```python
from build123d import *

# Parameters (mm, degrees)
PAD_DEPTH       = 41
SKETCH001_W     = 25
SKETCH001_H     = 50
POCKET_DEPTH    = 44.001
SKETCH002_W     = 45
SKETCH002_H     = 10
POCKET001_DEPTH = 30.001
SKETCH003_R     = 12
SKETCH003_R_2   = 1.625
POCKET002_DEPTH = 30.001
SKETCH004_R     = 2.75
POCKET003_DEPTH = 6.001
CHAMFER_SIZE    = 0.5
CHAMFER001_SIZE = 0.5
CHAMFER002_SIZE = 0.25


with BuildPart() as part:
    # Sketch → Pad (new body, symmetric)
    with BuildSketch(Plane.YZ):
        Polygon((0, 44), (0, 0), (-30, 0), (-30, 6), (-6, 44), align=None)
    extrude(amount=PAD_DEPTH, both=True)

    # Sketch001 → Pocket (cut, through all)
    with BuildSketch(Plane.YX):
        with Locations((-18.5, 0)):
            Rectangle(SKETCH001_W, SKETCH001_H)
    extrude(amount=-POCKET_DEPTH, mode=Mode.SUBTRACT)

    # Sketch002 → Pocket001 (cut, through all)
    with BuildSketch(Plane.ZX):
        with Locations((28.5, 36)):
            Rectangle(SKETCH002_W, SKETCH002_H)
        with Locations((28.5, -36)):
            Rectangle(SKETCH002_W, SKETCH002_H)
    extrude(amount=-POCKET001_DEPTH, mode=Mode.SUBTRACT)

    # Sketch003 → Pocket002 (cut, through all)
    with BuildSketch(Plane.ZX):
        with Locations((22, 0)):
            Circle(SKETCH003_R)
        with Locations((6.5, 15.5)):
            Circle(SKETCH003_R_2)
        with Locations((37.5, 15.5)):
            Circle(SKETCH003_R_2)
        with Locations((6.5, -15.5)):
            Circle(SKETCH003_R_2)
        with Locations((37.5, -15.5)):
            Circle(SKETCH003_R_2)
    extrude(amount=-POCKET002_DEPTH, mode=Mode.SUBTRACT)

    # Sketch004 → Pocket003 (cut, through all)
    with BuildSketch(Plane(origin=(0, 0, 6), x_dir=(0, -1, 0), z_dir=(0, 0, 1))):
        with Locations((5, 36)):
            Circle(SKETCH004_R)
        with Locations((25, 36)):
            Circle(SKETCH004_R)
        with Locations((5, -36)):
            Circle(SKETCH004_R)
        with Locations((25, -36)):
            Circle(SKETCH004_R)
    extrude(amount=-POCKET003_DEPTH, mode=Mode.SUBTRACT)

    # Chamfer
    chamfer_edges = [part.edges().sort_by_distance(p)[0] for p in [
        (36, -22.25, 6),
        (36, -2.25, 6),
        (-36, -22.25, 6),
        (-36, -2.25, 6),
    ]]
    chamfer(chamfer_edges, length=CHAMFER_SIZE)

    # Chamfer001
    chamfer001_edges = [part.edges().sort_by_distance(p)[0] for p in [
        (0, -6, 10),
        (0, 0, 10),
    ]]
    chamfer(chamfer001_edges, length=CHAMFER001_SIZE)

    # Chamfer002
    chamfer002_edges = [part.edges().sort_by_distance(p)[0] for p in [
        (15.5, 0, 35.875),
        (15.5, 0, 4.875),
        (-15.5, 0, 35.875),
        (-15.5, 0, 4.875),
        (15.5, -6, 35.875),
        (15.5, -6, 4.875),
        (-15.5, -6, 4.875),
        (-15.5, -6, 35.875),
    ]]
    chamfer(chamfer002_edges, length=CHAMFER002_SIZE)


solid = part.part
```
Geometry check sheet. Reference: the model listing, model coordinates, mm. A direction names the side the tool comes from. Give positions to 0.01 mm unless a question says otherwise; leave off trailing zeros. Order: outer loops, then holes, each group sorted by start corner. A loop starts at its lowest first (then second) coordinate and runs counter-clockwise, first axis right, second up. Notation, with made-up numbers: (-38, -33.5) - (-20, -33.5) arc R10 cw to (-20, -17.5) - close; hole circle Ø1 at (-1, 33). An arc over 180 degrees is marked (long way). Write item = value, one per line. Start each with the question number.
1) Section check B-B (z = 37.5). Enter the section's corners in (x, y) (3 decimals), then the cut area to 3 significant figures.
2) Draft check along Y on faces 6 (the cylindrical face through (-34.141, -22.973, 2.788)), 7 (the flat face through (28, -18, 25)), 8 (the flat face through (-36, -15, 6)), 9 (the cylindrical face through (38.727, -4.642, 2.788)). Enter one of: released by +Y, released by -Y, zero draft, split by the parting line, or undercut.
3) Gauge pin test, flat ends, axial feed: pin 1 Ø3 at (x, y) = (-37.5, -17) entering from +Z; pin 2 Ø3 at (x, z) = (-6, 14) entering from +Y; pin 3 Ø10 at (y, z) = (-8, 26) entering from -X; pin 4 Ø10 at (x, z) = (12, 25) entering from -Y. Record the tip position at first contact, or that the pin passes through.
4) Scan lines: L1, parallel to X at y = -25, z = 4.2; L2, parallel to X at y = -1.65, z = 6.5 (3 decimals); L3, parallel to X at y = -2, z = 37. Record each from-to range of solid material in increasing order.
5) Section check A-A (x = -15.5). Enter the section's corners in (y, z) (3 decimals), then the cut area to 3 significant figures.
6) Section check D-D (y = -25). Enter the section's corners in (x, z), then the cut area to 4 significant figures.
7) Access from +Z, -Z, +X, -X, +Y, -Y to the whole of each face (thin tool, end or side, straight path). Record for faces 1 (the flat face through (1, -5, 0)), 2 (the flat face through (-31, -11, 21)), 3 (the flat face through (25, -16, 17)), 4 (the flat face through (31, -11, 21)), 5 (the flat face through (41, -15, 3)).
8) Section check C-C (x = 0). Enter the section's corners in (y, z).
Geometry check:
q1.outline = (-31, -10.105) - (-25, -10.105) - (-25, -6) - (-17.375, -6) - (-17.125, -5.75) - (-17.125, -0.25) - (-17.375, 0) - (-31, 0) - close; (-13.875, -5.75) - (-13.625, -6) - (13.625, -6) - (13.875, -5.75) - (13.875, -0.25) - (13.625, 0) - (-13.625, 0) - (-13.875, -0.25) - close; (17.125, -5.75) - (17.375, -6) - (25, -6) - (25, -10.105) - (31, -10.105) - (31, 0) - (17.375, 0) - (17.125, -0.25) - close
q1.area = 382 mm2
q2.face_6 = undercut
q2.face_7 = released by -Y
q2.face_8 = zero draft
q2.face_9 = undercut
q3.pin_1 = 6
q3.pin_2 = through
q3.pin_3 = -31
q3.pin_4 = -6
q4.L1 = -41 to -38.75, -33.25 to -25, 25 to 33.25, 38.75 to 41
q4.L2 = -31 to -17.125, -13.875 to 13.875, 17.125 to 31
q4.L3 = -31 to -17.05, -13.95 to 13.95, 17.05 to 31
q5.outline = (-6, 0) - (0, 0) - (0, 4.625) - (-0.25, 4.875) - (-5.75, 4.875) - (-6, 4.625) - close; (-6, 8.375) - (-5.75, 8.125) - (-0.25, 8.125) - (0, 8.375) - (0, 35.625) - (-0.25, 35.875) - (-5.75, 35.875) - (-6, 35.625) - close; (-6, 39.375) - (-5.75, 39.125) - (-0.25, 39.125) - (0, 39.375) - (0, 44) - (-6, 44) - close
q5.area = 225 mm2
q6.outline = (-41, 0) - (-38.75, 0) - (-38.75, 5.5) - (-39.25, 6) - (-41, 6) - close; (-33.25, 0) - (-25, 0) - (-25, 13.92) - (-31, 13.92) - (-31, 6) - (-32.75, 6) - (-33.25, 5.5) - close; (25, 0) - (33.25, 0) - (33.25, 5.5) - (32.75, 6) - (31, 6) - (31, 13.92) - (25, 13.92) - close; (38.75, 0) - (41, 0) - (41, 6) - (39.25, 6) - (38.75, 5.5) - close
q6.area = 220.5 mm2
q7.face_1 = -Z, +X, -X, +Y, -Y
q7.face_2 = +Z, -X, +Y, -Y
q7.face_3 = +Z, -Z, -Y
q7.face_4 = +Z, +X, +Y, -Y
q7.face_5 = +Z, -Z, +X, +Y, -Y
q8.outline = (-6, 0) - (0, 0) - (0, 9.5) - (-0.5, 10) - (-5.5, 10) - (-6, 9.5) - close; (-6, 34.5) - (-5.5, 34) - (-0.5, 34) - (0, 34.5) - (0, 44) - (-6, 44) - close
